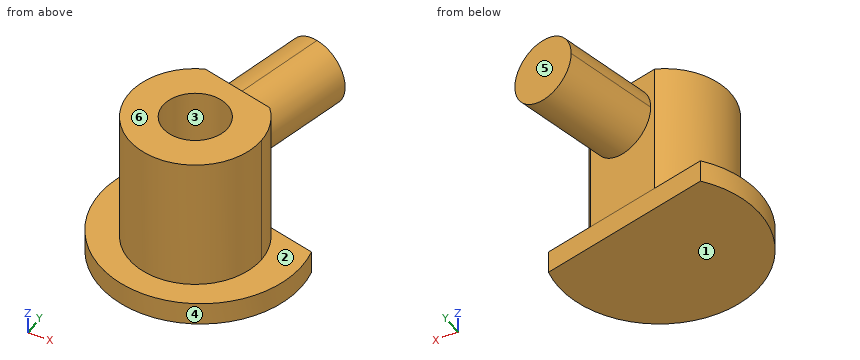
```python
from build123d import *

# Parameters (mm, degrees)
F1_DEPTH = 1.7
F2_R     = 2.4
F3_DEPTH = 10
F5_DEPTH = 7.5


with BuildPart() as f1:
    # F0 (on Top) → F1 (new body)
    with BuildSketch(Plane.XY):
        with BuildLine():
            Line((7.335345, 1.562919), (-5.774183, 4.786315))
            ThreePointArc((-5.774183, 4.786315), (-1.790775, -7.283071), (7.335345, 1.562919))
        make_face()
    extrude(amount=F1_DEPTH)

    # F2 (on face) → F3 (join)
    with BuildSketch(Plane.XY.offset(1.7)):
        with BuildLine():
            ThreePointArc((-1.825206, 3.815333), (-2.744676, -4.791199), (4.9, -0.732042))
            ThreePointArc((4.9, -0.732042), (4.597097, 0.964042), (3.725836, 2.450432))
            Line((3.725836, 2.450432), (-1.825206, 3.815333))
        make_face()
        with Locations((0, -0.732042)):
            Circle(F2_R, mode=Mode.SUBTRACT)
    extrude(amount=F3_DEPTH)

    # F4 (on face) → F5 (join)
    with BuildSketch(Plane(origin=(0.780581, 3.174617, 0), x_dir=(-0.971076, 0.23877, 0), z_dir=(0.23877, 0.971076, 0))):
        with BuildLine():
            ThreePointArc((2.32521, 8.7), (1.592977, 10.467767), (-0.17479, 11.2))
            ThreePointArc((-0.17479, 11.2), (-1.942557, 6.932233), (2.32521, 8.7))
        make_face()
    extrude(amount=F5_DEPTH)


solid = f1.part
```
Input: part model. Units: mm. Frame: model coordinates. Face numbers are marked on the shaded views. A direction names the side the tool comes from. Round coordinates to 2 decimals unless told otherwise and drop trailing zeros. Write each loop counter-clockwise with the first axis right and the second up, starting at its lowest first coordinate (ties: lowest second). Pieces come first, ordered by that corner, then holes. Notation, with made-up numbers: (-4.5, 50) -> (0.5, 50) arc R7 ccw to (0.5, 56) -> close; hole circle Ø1 at (86.25, -38). An arc over 180 degrees is marked (long way). Answer as CSV lines item,"result".
1. Ray query, L1, parallel to Z at x = 0.75, y = -5.75; L2, parallel to X at y = -4.5, z = 4.5; L3, parallel to X at y = 1, z = 2. Return the intervals inside material, ascending. Write a range as [from, to].
Geometry says:
L1,"z = [0, 1.7]"
L2,"x = [-3.13, 3.13]"
L3,"x = [-4.58, -1.66], [1.66, 4.58]"
2. Section B-B (y = -0.25). Return the cut outline in (x, z), plus the area to 3 significant figures.
Geometry says:
outline,"(-7.5, 0) -> (7.5, 0) -> (7.5, 1.7) -> (4.88, 1.7) -> (4.88, 11.7) -> (2.35, 11.7) -> (2.35, 1.7) -> (-2.35, 1.7) -> (-2.35, 11.7) -> (-4.88, 11.7) -> (-4.88, 1.7) -> (-7.5, 1.7) -> close"
area,"76.0 mm^2"
3. Section A-A (z = 2.25). Return the cut outline in (x, y), plus the area to 3 significant figures.
Geometry says:
outline,"(-1.83, 3.82) arc R4.9 ccw (long way) to (4.9, -0.73) arc R4.9 ccw to (3.73, 2.45) -> close; hole circle Ø4.8 at (0, -0.73)"
area,"53.8 mm^2"
4. Section C-C (z = 8). Return the cut outline in (x, y), plus the area to 3 significant figures.
Geometry says:
outline,"(-1.83, 3.82) arc R4.9 ccw (long way) to (4.9, -0.73) arc R4.9 ccw to (3.73, 2.45) -> (3.28, 2.56) -> (5.07, 9.84) -> (0.41, 10.99) -> (-1.38, 3.71) -> close; hole circle Ø4.8 at (0, -0.73)"
area,"89.8 mm^2"
5. Contact query for flat-ended pins moving along their axis: P1, Ø5, axis at y = 8.5, z = 4.5, coming from the -X side; P2, Ø1.5, axis at x = 1, y = 8.5, coming from the +Z side; P3, Ø1.4, axis at x = 1, y = -0.5, coming from the +Z side. Output: stop coordinate, or through.
Geometry says:
P1,"stops at x = 0.31"
P2,"stops at z = 11.15"
P3,"stops at z = 1.7"
6. Mould query, pull axis Y, two halves, no side actions, for the marked faces 3, 4, 5 and 6. Classes: +Y half, -Y half, draft (parallel to the pull), parting line (faces both ways), or undercut.
Geometry says:
face 3,"undercut"
face 4,"parting line"
face 5,"+Y half"
face 6,"draft"
7. Reachability of the marked faces 1 and 2 from +Z, -Z, +X, -X, +Y, -Y: full face, straight path, thin tool, end or side. Return the list, or none.
Geometry says:
face 1,"-Z, +X, -X, +Y, -Y"
face 2,"+Z"
